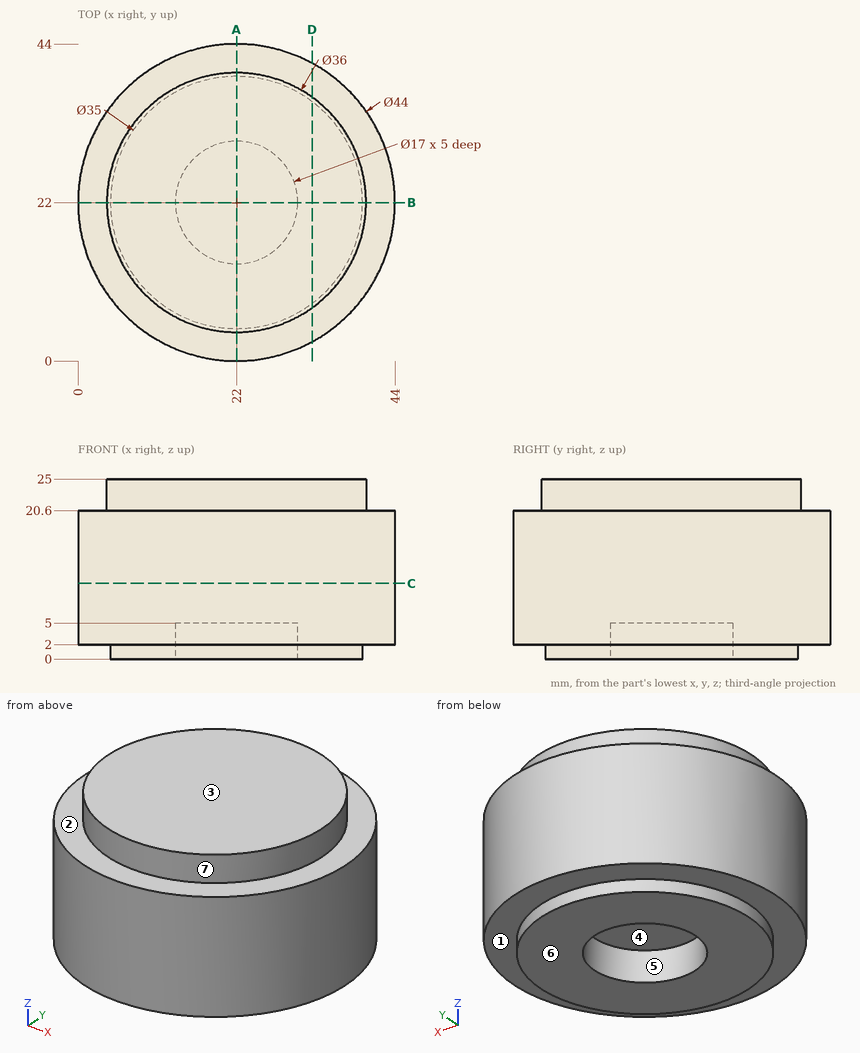
Study the drawing (mm; zero at the part's minimum x, y, z) and answer. A direction names the side the tool comes from. Give positions to 0.01 mm unless a question says otherwise; leave off trailing zeros. Write each loop counter-clockwise with the first axis right and the second up, starting at its lowest first coordinate (ties: lowest second). Pieces come first, ordered by that corner, then holes. Notation, with made-up numbers: (71, 54.25) -> (75, 54.25) arc R33 ccw to (75, 88.25) -> close; hole circle Ø2 at (69, 61). An arc over 180 degrees is marked (long way). Answer in a Markdown table with one row per item.
1) Section C-C on z = 10.5 is taken. Give the vertices of the cut face in (x, y).
Results list:
| item | result |
|---|---|
| outline | circle Ø44 at (22, 22) |
2) Straight lines are drawn through the part: line 1 (Y direction, x = 22, z = 2.2); line 2 (Y direction, x = 22, z = 1.25); line 3 (Z direction, x = 23.5, y = 4.5). For each, find the intervals that lie inside material, in ascending order. Write a range as [from, to].
Results list:
| item | result |
|---|---|
| line 1 | [0, 13.5], [30.5, 44] |
| line 2 | [4.5, 13.5], [30.5, 39.5] |
| line 3 | [2, 25] |
3) Each of these flat-tipped pins is pushed along its axis until it touches: pin 1 Ø3 at (x, z) = (15.5, 15) entering from -Y; pin 2 Ø1.5 at (x, z) = (8.5, 19) entering from -Y; pin 3 Ø5 at (x, y) = (30.5, 27.5) entering from -Z; pin 4 Ø6 at (x, z) = (6.5, 18.5) entering from +Y. Where does it stop, or does it pass through?
Results list:
| item | result |
|---|---|
| pin 1 | y = 0.58 |
| pin 2 | y = 4.07 |
| pin 3 | z = 0 |
| pin 4 | y = 40.1 |
4) Determine the mould class of the marked faces 4, 5, 6 and 7 for opening direction Y: released by +Y, released by -Y, zero draft, split by the parting line, or undercut.
Results list:
| item | result |
|---|---|
| face 4 | undercut |
| face 5 | undercut |
| face 6 | zero draft |
| face 7 | split by the parting line |
5) Section D-D on x = 32.5 is taken. Give the vertices of the cut face in (y, z).
Results list:
| item | result |
|---|---|
| outline | (2.67, 2) -> (8, 2) -> (8, 0) -> (36, 0) -> (36, 2) -> (41.33, 2) -> (41.33, 20.6) -> (36.62, 20.6) -> (36.62, 25) -> (7.38, 25) -> (7.38, 20.6) -> (2.67, 20.6) -> close |
6) A tool of negligible diameter and unlimited length cuts with its end or side. For the marked faces 1, 2 and 3, from which of +Z, -Z, +X, -X, +Y, -Y can it reach the whole face along a straight path? Write none if from no direction.
Results list:
| item | result |
|---|---|
| face 1 | -Z |
| face 2 | +Z |
| face 3 | +Z, +X, -X, +Y, -Y |
7) Section A-A on x = 22 is taken. Give the vertices of the cut face in (y, z), plus the area to 3 significant figures.
Results list:
| item | result |
|---|---|
| outline | (0, 2) -> (4.5, 2) -> (4.5, 0) -> (13.5, 0) -> (13.5, 5) -> (30.5, 5) -> (30.5, 0) -> (39.5, 0) -> (39.5, 2) -> (44, 2) -> (44, 20.6) -> (40, 20.6) -> (40, 25) -> (4, 25) -> (4, 20.6) -> (0, 20.6) -> close |
| area | 962 mm^2 |
